Geometry: final body of the model. Coordinates: model frame, mm. A direction names the side the tool comes from. Round coordinates to 2 decimals unless told otherwise and drop trailing zeros. Order: outer loops, then holes, each group sorted by start corner. A loop starts at its lowest first (then second) coordinate and runs counter-clockwise, first axis right, second up. Notation, with made-up numbers: (80.5, -39) -> (131.5, -39) arc R13 cw to (131.5, -25) -> close; hole circle Ø2 at (62.25, 84.5). An arc over 180 degrees is marked (long way). Put each result on its own line as item: value.
```python
from build123d import *

# Parameters (mm, degrees)
F1_DEPTH = 63.5
F2_DEPTH = 25.4
F3_DEPTH = 25.4
F4_DEPTH = 7.9375
F6_R     = 6.35


with BuildPart() as f1:
    # F0 (on Front) → F1 (new body, symmetric)
    with BuildSketch(Plane.XZ):
        Polygon((-41.275, 9.525), (-41.275, -9.525), (41.275, -9.525), (41.275, 9.525), (22.2250011172, 9.525), align=None)
    extrude(amount=F1_DEPTH, both=True)

    # F0 (on Front) → F2 (join, symmetric)
    with BuildSketch(Plane.XZ):
        with BuildLine():
            Line((22.2250011172, 9.525), (41.275, 9.525))
            Line((41.275, 9.525), (41.275, 27.0002))
            ThreePointArc((41.275, 27.0002), (45.9246798487, 38.2255201513), (57.15, 42.8752))
            Line((57.15, 42.8752), (60.325, 42.8752))
            Line((60.325, 42.8752), (60.325, 61.9251988828))
            Line((60.325, 61.9251988828), (57.15, 61.9251988828))
            add(Edge.make_bspline(
                [(55.4567430493, 61.8841279306), (56.0220700945, 61.8996898871), (56.5865253234, 61.913371712), (57.15, 61.9251988828)],
                knots=[110.1217614603, 110.1217614603, 110.1217614603, 110.1217614603, 111.5045356385, 111.5045356385, 111.5045356385, 111.5045356385], degree=3))
            ThreePointArc((55.4567430493, 61.8841279306), (31.8627250966, 51.089809273), (22.2250011172, 27.0002))
            Line((22.2250011172, 27.0002), (22.2250011172, 9.525))
        make_face()
    extrude(amount=F2_DEPTH, both=True)

    # F3 (add): a face of the model
    f3_faces = [f1.faces().sort_by_distance(p)[0] for p in [
        (60.325, 0, 52.4001994414),
    ]]
    extrude(f3_faces, amount=F3_DEPTH)

    # F0 (on Front) → F4 (join, symmetric)
    with BuildSketch(Plane.XZ):
        with BuildLine():
            add(Edge.make_bspline(
                [(-41.275, 9.525), (-40.1158891468, 47.4811966341), (10.4350677867, 60.6448004288), (55.4567430493, 61.8841279306)],
                knots=[0, 0, 0, 0, 110.1217614603, 110.1217614603, 110.1217614603, 110.1217614603], degree=3))
            Line((-41.275, 9.525), (22.2250011172, 9.525))
            Line((22.2250011172, 9.525), (22.2250011172, 27.0002))
            ThreePointArc((22.2250011172, 27.0002), (31.8627250966, 51.089809273), (55.4567430493, 61.8841279306))
        make_face()
    extrude(amount=F4_DEPTH, both=True)

    # F0 (on Front) → F5 (revolve)
    with BuildSketch(Plane.XZ):
        Polygon((111.125, 66.675), (76.2634606961, 66.675), (76.2987583876, 38.1), (111.125, 38.1), align=None)
    revolve(axis=Axis((76.2811095418, 0, 52.3875), (-0.0012352639, 0, 0.9999992371)))

    # F6
    f6_edges = [f1.edges().sort_by_distance(p)[0] for p in [
        (-41.275, -63.5, 0),
        (41.275, -63.5, 0),
        (41.275, 63.5, 0),
        (-41.275, 63.5, 0),
    ]]
    fillet(f6_edges, radius=F6_R)


solid = f1.part
```
1. Set-up query: faces 1 (the face through (-1, -1, -9.525)), 2 (the face through (37, 25.4, 35)), 3 (the face through (27.706, -16.791, 45.784)), 4 (the face through (41.275, -1, 4)). Return all of +Z, -Z, +X, -X, +Y, -Y with unobstructed straight access to the full face (end or side cutting, diameter ignored); none if empty.
Ans:
face 1: -Z, +X, -X, +Y, -Y
face 2: +Z, -X, +Y
face 3: +Z, -X, -Y
face 4: -Z, +X, +Y, -Y
2. Cut plane B-B on y = 46. Return loops of the section in (x, z) (3 decimals), and give its area (3 significant figures).
Ans:
outline: (-41.275, -9.525) -> (41.275, -9.525) -> (41.275, 9.525) -> (-41.275, 9.525) -> close
area: 1,570 mm²
3. Contact query for flat-ended pins moving along their axis: P1, Ø1, axis at x = 89.5, y = 1.5, coming from the -Z side; P2, Ø4, axis at x = 20.5, y = -27, coming from the +Z side (3 decimals); P3, Ø8, axis at x = 45, y = 4, coming from the +Z side; P4, Ø1, axis at y = 34.5, z = 37, coming from the +X side. Output: stop coordinate, or through.
Ans:
P1: z = 38.1
P2: z = 9.525
P3: z = 66.61
P4: through
4. Material intervals for probe 1 along X at (y, z) = (44, 3.5) (3 decimals); probe 2 along Z at (x, y) = (-22, -25.5) (3 decimals); probe 3 along X at (y, z) = (-10.5, 12.5) (3 decimals), sorted ascending.
Ans:
probe 1: -41.275 to 41.275
probe 2: -9.525 to 9.525
probe 3: 22.225 to 41.275
5. Cut plane A-A on z = 5.5. Return loops of the section in (x, y) (3 decimals), and give its area (3 significant figures).
Ans:
outline: (-41.275, -57.15) arc R6.35 ccw to (-34.925, -63.5) -> (34.925, -63.5) arc R6.35 ccw to (41.275, -57.15) -> (41.275, 57.15) arc R6.35 ccw to (34.925, 63.5) -> (-34.925, 63.5) arc R6.35 ccw to (-41.275, 57.15) -> close
area: 10,400 mm²
